Geometry: final body of the model. Coordinates: model frame, mm. Face numbers are marked on the shaded views. Give positions to 0.01 mm unless a question says otherwise; leave off trailing zeros. Write each loop counter-clockwise with the first axis right and the second up, starting at its lowest first coordinate (ties: lowest second). Pieces come first, ordered by that corner, then holes.
Q1. Cut plane A-A on z = 4.5. Return the cut outline in (x, y) (3 decimals).
Q2. Draft query along Z for the marked faces 1, 2 and 3. Return one class per face: pulls with the +Z half, pulls with the -Z half, needs draft (parallel to the pull), parting line crosses it, or undercut.
Q3. Cut plane B-B on z = 21.75. Return the cut outline in (x, y) (3 decimals).
Q4. Pin query (flat end, axial travel): pin 1 (10 mm diameter, centred on x = 9, z = 15, fed in from -Y); pin 2 (3.5 mm diameter, centred on x = -7.5, y = 5, fed in from +Z) (3 decimals). Return the tip coordinate at first contact, or that it passes through.
Q5. Line query: L1, parallel to X at y = -0.5, z = 5.75 (3 decimals); L2, parallel to Z at x = 5.5, y = 3 (3 decimals); L3, parallel to X at y = 9, z = 5 (3 decimals). Output: solid intervals per line, ascending.
```python
from build123d import *

# Parameters (mm, degrees)
F1_DEPTH = 25.4
F2_R     = 12.7
F3_DEPTH = 3.175
F5_DEPTH = 12.7
F6_SIZE2 = 1.4566665597
F6_SIZE  = 5.08


with BuildPart() as f1:
    # F0 (on Top) → F1 (new body)
    with BuildSketch(Plane.XY):
        with BuildLine():
            ThreePointArc((-15.875, 0), (-11.2253201513, 11.2253201513), (0, 15.875))
            Line((0, 15.875), (-15.875, 15.875))
            Line((-15.875, 15.875), (-15.875, 0))
        make_face()
        with BuildLine():
            Line((-15.875, -15.875), (0, -15.875))
            ThreePointArc((0, -15.875), (-11.2253201513, -11.2253201513), (-15.875, 0))
            Line((-15.875, 0), (-15.875, -15.875))
        make_face()
        with BuildLine():
            Line((0, -15.875), (0, -12.7))
            ThreePointArc((0, -12.7), (-8.9802561211, -8.9802561211), (-12.7, 0))
            Line((-12.7, 0), (-15.875, 0))
            ThreePointArc((-15.875, 0), (-11.2253201513, -11.2253201513), (0, -15.875))
        make_face()
        with BuildLine():
            ThreePointArc((-12.7, 0), (-8.9802561211, 8.9802561211), (0, 12.7))
            Line((0, 12.7), (0, 15.875))
            ThreePointArc((0, 15.875), (-11.2253201513, 11.2253201513), (-15.875, 0))
            Line((-15.875, 0), (-12.7, 0))
        make_face()
        with BuildLine():
            ThreePointArc((0, 12.7), (8.9802561211, 8.9802561211), (12.7, 0))
            ThreePointArc((12.7, 0), (8.9802561211, -8.9802561211), (0, -12.7))
            Line((0, -12.7), (0, -15.875))
            ThreePointArc((0, -15.875), (11.2253201513, -11.2253201513), (15.875, 0))
            ThreePointArc((15.875, 0), (11.2253201513, 11.2253201513), (0, 15.875))
            Line((0, 15.875), (0, 12.7))
        make_face()
    extrude(amount=F1_DEPTH)

    # F2 (on face) → F3 (join)
    with BuildSketch(Plane(origin=(0, 0, 0), x_dir=(1, 0, 0), z_dir=(0, 0, -1))):
        with BuildLine():
            Line((-15.875, 15.875), (-15.875, -15.875))
            Line((-15.875, -15.875), (0, -15.875))
            ThreePointArc((0, -15.875), (15.875, 0), (0, 15.875))
            Line((0, 15.875), (-15.875, 15.875))
        make_face()
        Circle(F2_R, mode=Mode.SUBTRACT)
        Circle(F2_R)
    extrude(amount=-F3_DEPTH)

    # F4 (on face) → F5 (cut)
    with BuildSketch(Plane(origin=(-15.875, 0, 0), x_dir=(0, -1, 0), z_dir=(-1, 0, 0))):
        Polygon((0, 6.35), (0, 9.525), (-7.9375, 9.525), (-11.90625, 9.525), (-11.90625, 6.35), (-7.9375, 6.35), align=None)
        Polygon((7.9375, 9.525), (0, 9.525), (0, 6.35), (7.9375, 6.35), (11.90625, 6.35), (11.90625, 9.525), align=None)
    extrude(amount=-F5_DEPTH, mode=Mode.SUBTRACT)

    # F6
    f6_edges = [f1.edges().sort_by_distance(p)[0] for p in [
        (0, -12.7, 25.4),
    ]]
    f6_side = f1.faces().sort_by_distance((0, -12.7, 14.2875))[0]
    chamfer(f6_edges, length=F6_SIZE, length2=F6_SIZE2, reference=f6_side)


solid = f1.part
```
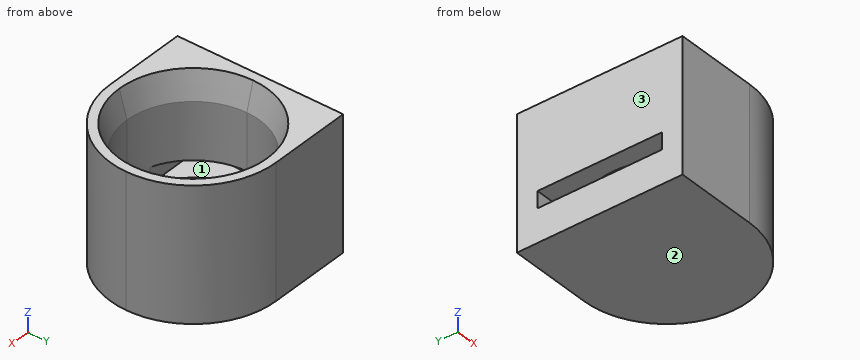
Data:
1. outline: (-15.875, -15.875) - (0, -15.875) arc R15.875 ccw to (0, 15.875) - (-15.875, 15.875) - close; hole circle Ø25.4 at (0, 0)
2. face 1: undercut
2. face 2: pulls with the -Z half
2. face 3: needs draft
3. outline: (-15.875, -15.875) - (0, -15.875) arc R15.875 ccw to (0, 15.875) - (-15.875, 15.875) - close; hole circle Ø26.22 at (0, 0)
4. pin 1: stops at y = -15.36
4. pin 2: stops at z = 3.175
5. L1: x = -15.875 to -12.69, 12.69 to 15.867
5. L2: z = 0 to 3.175
5. L3: x = -15.875 to -8.96, 8.96 to 13.077
